Could you check a few things on this model? Use its own coordinates, in mm. A direction names the side the tool comes from. Give positions to 0.01 mm unless a question says otherwise; leave off trailing zeros. Order: outer loops, then holes, each group sorted by start corner. A loop starts at its lowest first (then second) coordinate and runs counter-clockwise, first axis right, second up.
from build123d import *

# Parameters (mm, degrees)
F0_W     = 80
F0_H     = 80
F1_DEPTH = 51.5
F2_T     = -1.5
F4_DEPTH = 50
F5_W     = 3
F5_H     = 1.5
F6_DEPTH = 1.5


with BuildPart() as f1:
    # F0 (on Top) → F1 (new body)
    with BuildSketch(Plane.XY):
        Rectangle(F0_W, F0_H)
    extrude(amount=F1_DEPTH)

    # F2
    f2_openings = [f1.faces().sort_by_distance(p)[0] for p in [
        (0, 0, 51.5),
    ]]
    offset(amount=F2_T, openings=f2_openings)

    # F3 (on face) → F4 (join, through all)
    with BuildSketch(Plane.XY.offset(51.5)):
        with BuildLine():
            ThreePointArc((-36.9999999833, 38.5), (-35.9393398223, 38.0606601659), (-35.5, 37))
            ThreePointArc((-35.5, 37), (-37, 35.5), (-38.5, 37))
            Line((-38.5, 37), (-38.5, 34))
            Line((-38.5, 34), (-37, 34))
            ThreePointArc((-37, 34), (-34.8786796564, 34.8786796564), (-34, 37))
            Line((-34, 37), (-34, 38.5))
            Line((-34, 38.5), (-36.9999999833, 38.5))
        make_face()
        with BuildLine():
            ThreePointArc((-38.5, 37), (-38.0606601659, 38.0606601777), (-36.9999999833, 38.5))
            Line((-36.9999999833, 38.5), (-38.5, 38.5))
            Line((-38.5, 38.5), (-38.5, 37))
        make_face()
        with BuildLine():
            Line((-37, -34), (-38.5, -34))
            Line((-38.5, -34), (-38.5, -37))
            ThreePointArc((-38.5, -37), (-37, -35.5), (-35.5, -37))
            ThreePointArc((-35.5, -37), (-35.9393398378, -38.0606601813), (-37.0000000271, -38.5))
            Line((-37.0000000271, -38.5), (-34, -38.5))
            Line((-34, -38.5), (-34, -37))
            ThreePointArc((-34, -37), (-34.8786796564, -34.8786796564), (-37, -34))
        make_face()
        with BuildLine():
            ThreePointArc((-37.0000000271, -38.5), (-38.0606601813, -38.0606601622), (-38.5, -37))
            Line((-38.5, -37), (-38.5, -38.5))
            Line((-38.5, -38.5), (-37.0000000271, -38.5))
        make_face()
        with BuildLine():
            Line((38.5, -37), (38.5, -34))
            Line((38.5, -34), (37, -34))
            ThreePointArc((37, -34), (34.8786796564, -34.8786796564), (34, -37))
            Line((34, -37), (34, -38.5))
            Line((34, -38.5), (37, -38.5))
            ThreePointArc((37, -38.5), (35.9393398282, -35.9393398282), (38.5, -37))
        make_face()
        with BuildLine():
            Line((38.5, -38.5), (38.5, -37))
            ThreePointArc((38.5, -37), (38.0606601718, -38.0606601718), (37, -38.5))
            Line((37, -38.5), (38.5, -38.5))
        make_face()
        with BuildLine():
            Line((37.0000000167, 38.5), (34, 38.5))
            Line((34, 38.5), (34, 37))
            ThreePointArc((34, 37), (34.8786796564, 34.8786796564), (37, 34))
            Line((37, 34), (38.5, 34))
            Line((38.5, 34), (38.5, 37))
            ThreePointArc((38.5, 37), (35.9393398223, 35.9393398341), (37.0000000167, 38.5))
        make_face()
        with BuildLine():
            Line((38.5, 38.5), (37.0000000167, 38.5))
            ThreePointArc((37.0000000167, 38.5), (38.0606601777, 38.0606601659), (38.5, 37))
            Line((38.5, 37), (38.5, 38.5))
        make_face()
    extrude(amount=-F4_DEPTH)

    # F5 (on face) → F6 (cut, through all)
    with BuildSketch(Plane.XZ.offset(40)):
        with Locations((0, 3.75)):
            Rectangle(F5_W, F5_H)
    extrude(amount=-F6_DEPTH, mode=Mode.SUBTRACT)


solid = f1.part
Item 1: For faces 4 (the flat face through (38.5, 0, 26)), 5 (the flat face through (-40, -1, 25)), which set-ups out of +Z, -Z, +X, -X, +Y, -Y let a thin tool reach every point of the face, with its end or its side?
Findings:
face 4: +Z
face 5: +Z, -Z, -X, +Y, -Y
Item 2: Imagine slicing it at B-B on y = 9.5. List the corners of the cut face in (x, z) for me.
Findings:
outline: (-40, 0) - (40, 0) - (40, 51.5) - (38.5, 51.5) - (38.5, 1.5) - (-38.5, 1.5) - (-38.5, 51.5) - (-40, 51.5) - close
Item 3: For pin 1 (4 mm diameter, centred on x = 8, y = 19, fed in from +Z), with a flat end and sliding along its axis, tell me the tip position at first contact or that it passes through.
Findings:
pin 1: stops at z = 1.5
Item 4: Please list where these lines run through material, in increasing order: line 1 along X through (y, z) = (37, 37.5); line 2 along Y through (x, z) = (29, 12).
Findings:
line 1: x = -40 to -38.5, -35.5 to -34, 34 to 35.5, 38.5 to 40
line 2: y = -40 to -38.5, 38.5 to 40
Item 5: We'd pull the mould along X, two halves only. Please class faces 1 (the flat face through (40, -1, 25)), 2 (the flat face through (-1, 1, 0)), 3 (the flat face through (-37, 37, 1.5)): +X half, -X half, draft (parallel to the pull), parting line (faces both ways), or undercut.
Findings:
face 1: +X half
face 2: draft
face 3: undercut
Item 6: Imagine slicing it at A-A on z = 10. List the corners of the cut face in (x, y) for me.
Findings:
outline: (-40, -40) - (40, -40) - (40, 40) - (-40, 40) - close; hole circle Ø3 at (-37, -37); hole (-38.5, -34) - (-37, -34) arc R3 cw to (-34, -37) - (-34, -38.5) - (34, -38.5) - (34, -37) arc R3 cw to (37, -34) - (38.5, -34) - (38.5, 34) - (37, 34) arc R3 cw to (34, 37) - (34, 38.5) - (-34, 38.5) - (-34, 37) arc R3 cw to (-37, 34) - (-38.5, 34) - close; hole circle Ø3 at (-37, 37); hole circle Ø3 at (37, -37); hole circle Ø3 at (37, 37)
